Could you check a few things on this model? Use its own coordinates, in mm. A direction names the side the tool comes from. Round coordinates to 2 decimals unless told otherwise and drop trailing zeros. Write each loop counter-clockwise with the first axis right and the second up, starting at its lowest first coordinate (ties: lowest second). Pieces come first, ordered by that corner, then holes. Notation, with made-up numbers: (-31.5, 78) -> (-12.5, 78) arc R28 ccw to (-12.5, 112) -> close; hole circle Ø4 at (71, 82.25). An arc over 180 degrees is marked (long way). Answer in a Markdown table with one row per item.
from build123d import *

# Parameters (mm, degrees)
SHELL_1_T                = -4.4
SKETCH_4_W               = 30
SKETCH_4_H               = 20
CUT_EXTRUDE_2_DEPTH      = 143.273012367
FILLET_1_R               = 2
SKETCH_6_W               = 23
SKETCH_6_H               = 12.5
EXTRUDE_1_DEPTH          = 5.5
SKETCH_7_R               = 1.5
CUT_EXTRUDE_3_DEPTH      = 147.482115115
SKETCH_8_R               = 1.6
CUT_EXTRUDE_4_DEPTH      = 2.2
CUT_EXTRUDE_1_DEPTH      = 3.4
CUT_EXTRUDE_START        = -3.4
CUT_EXTRUDE_5_DEPTH      = 3.4
CUT_EXTRUDE_6_DEPTH      = 154.574086519
CUT_EXTRUDE_6_DEPTH_BACK = 154.574086519
SKETCH_10_R              = 2.75
SKETCH_11_R              = 3
EXTRUDE_2_DEPTH          = 3
HOLE_WIZARD_M3_1_D       = 3.4
HOLE_WIZARD_M3_1_DEPTH   = 4.4001
EXTRUDE_3_DEPTH          = 3


with BuildPart() as part:
    # 草图1 → 放样1 section 0
    with BuildSketch(Plane(origin=(0, 0, 0), x_dir=(1, 0, 0), z_dir=(0, 1, 0))):
        with BuildLine():
            Line((-62.5, 55), (62.5, 55))
            Line((62.5, 55), (62.5, -55))
            Line((62.5, -55), (-62.5, -55))
            Line((-62.5, -55), (-62.5, 55))
        make_face()
    # 草图2 → 放样1 section 1
    with BuildSketch(Plane(origin=(0, 72, 0), x_dir=(1, 0, 0), z_dir=(0, 1, 0))):
        with BuildLine():
            Line((-62.5, 55), (62.5, 55))
            Line((62.5, 55), (62.5, -55))
            Line((62.5, -55), (-62.5, -55))
            Line((-62.5, -55), (-62.5, 55))
        make_face()
    loft()

    # 抽壳1
    shell_1_openings = [part.faces().sort_by_distance(p)[0] for p in [
        (0, 72, 0),
    ]]
    offset(amount=SHELL_1_T, openings=shell_1_openings, kind=Kind.INTERSECTION)

    # 草图4 → 切除-拉伸2 (cut, through all)
    with BuildSketch(Plane.XY.offset(50.6)):
        with Locations((-22.217899847, 24.659135412)):
            Rectangle(SKETCH_4_W, SKETCH_4_H)
    extrude(amount=CUT_EXTRUDE_2_DEPTH, mode=Mode.SUBTRACT)

    # 圆角1
    fillet_1_edges = [part.edges().sort_by_distance(p)[0] for p in [
        (-7.217899847, 14.659135412, 52.8),
        (-7.217899847, 34.659135412, 52.8),
        (-37.217899847, 34.659135412, 52.8),
        (-37.217899847, 14.659135412, 52.8),
    ]]
    fillet(fillet_1_edges, radius=FILLET_1_R)

    # 草图6 → 凸台-拉伸1 (add)
    with BuildSketch(Plane(origin=(-58.1, 0, 0), x_dir=(0, 0, -1), z_dir=(1, 0, 0))):
        Polygon((-21.75, 42.25), (-21.75, 47.25), (11.25, 47.25), (11.25, 42.25), (11.25, 29.74999898), (11.25, 24.75), (-21.75, 24.75), (-21.75, 29.74999898), align=None)
        with Locations((-5.25, 36)):
            Rectangle(SKETCH_6_W, SKETCH_6_H, mode=Mode.SUBTRACT)
    extrude_1 = extrude(amount=EXTRUDE_1_DEPTH)

    # 草图7 → 切除-拉伸3 (cut, through all)
    with BuildSketch(Plane(origin=(-52.6, 0, 0), x_dir=(0, 0, -1), z_dir=(1, 0, 0))):
        with Locations(Location((-19, 35.99999884, 0), (0, 0, 90))):
            Circle(SKETCH_7_R)
        with Locations(Location((8.5, 35.99999884, 0), (0, 0, 90))):
            Circle(SKETCH_7_R)
    cut_extrude_3 = extrude(amount=-CUT_EXTRUDE_3_DEPTH, mode=Mode.SUBTRACT)

    # 镜向1: 凸台-拉伸1, 切除-拉伸3 across plane
    add(extrude_1.mirror(Plane(origin=(0, 0, 0), x_dir=(0, 0, 1), z_dir=(1, 0, 0))))
    add(cut_extrude_3.mirror(Plane(origin=(0, 0, 0), x_dir=(0, 0, 1), z_dir=(1, 0, 0))), mode=Mode.SUBTRACT)

    # 草图8 → 切除-拉伸4 (cut)
    with BuildSketch(Plane(origin=(0, 72, 0), x_dir=(1, 0, 0), z_dir=(0, 1, 0))):
        with Locations(Location((-60, 52.5, 0), (0, 0, 270))):
            Circle(SKETCH_8_R)
        with Locations(Location((-60, -52.5, 0), (0, 0, 270))):
            Circle(SKETCH_8_R)
        with Locations(Location((60, -52.5, 0), (0, 0, 270))):
            Circle(SKETCH_8_R)
        with Locations(Location((60, 52.5, 0), (0, 0, 270))):
            Circle(SKETCH_8_R)
    extrude(amount=-CUT_EXTRUDE_4_DEPTH, mode=Mode.SUBTRACT)

    # 草图3 → 切除-拉伸1 (cut)
    with BuildSketch(Plane(origin=(-58.1, 0, 0), x_dir=(0, 0, -1), z_dir=(1, 0, 0))):
        with BuildLine():
            ThreePointArc((-5.75, 38.449489743), (-8.75, 36), (-5.75, 33.550510257))
            ThreePointArc((-5.75, 33.550510257), (6.25, 36), (-5.75, 38.449489743))
        make_face()
    extrude(amount=-CUT_EXTRUDE_1_DEPTH, mode=Mode.SUBTRACT)

    # 草图9 → 切除-拉伸5 (cut)
    with BuildSketch(Plane.ZY.offset(-58.1).offset(CUT_EXTRUDE_START)):
        with BuildLine():
            ThreePointArc((5.75, 38.449489743), (-6.25, 36), (5.75, 33.550510257))
            ThreePointArc((5.75, 33.550510257), (8.75, 36), (5.75, 38.449489743))
        make_face()
    extrude(amount=CUT_EXTRUDE_5_DEPTH, mode=Mode.SUBTRACT)

    # 草图10 → 切除-拉伸6 (cut, two sides: drawn at the far end of the back side and taken through both)
    with BuildSketch(Plane(origin=(-61.5, 0, 0), x_dir=(0, 0, -1), z_dir=(1, 0, 0)).offset(-CUT_EXTRUDE_6_DEPTH_BACK)):
        with Locations(Location((0, 36, 0), (0, 0, 270))):
            Circle(SKETCH_10_R)
    extrude(amount=CUT_EXTRUDE_6_DEPTH + CUT_EXTRUDE_6_DEPTH_BACK, mode=Mode.SUBTRACT)

    # 草图11 → 凸台-拉伸2 (add)
    with BuildSketch(Plane(origin=(0, 0, -55), x_dir=(-1, 0, 0), z_dir=(0, 0, -1))):
        with Locations(Location((42.5, 24.543593294, 0), (0, 0, 270))):
            Circle(SKETCH_11_R)
        with Locations(Location((24.5, 24.543593294, 0), (0, 0, 270))):
            Circle(SKETCH_11_R)
    extrude(amount=EXTRUDE_2_DEPTH)

    # M3 间隙孔1
    with Locations(Plane(origin=(0, 0, 50.6), x_dir=(-1, 0, 0), z_dir=(0, 0, -1))):
        with Locations((-40.5, 63.5), (0, 63.5), (40.5, 63.5), (40.5, 36), (-40.5, 36)):
            Hole(HOLE_WIZARD_M3_1_D / 2, depth=HOLE_WIZARD_M3_1_DEPTH)

    # 草图15 → 凸台-拉伸3 (add)
    with BuildSketch(Plane(origin=(0, 0, 50.6), x_dir=(-1, 0, 0), z_dir=(0, 0, -1))):
        Polygon((-29.1, 60.00000762), (-29.1, 58), (-33.10001016, 58), (-33.10001016, 57), (-28.112700025, 57), (-28.1, 60.00000762), align=None)
        Polygon((-4.825356871, 58), (-4.825356871, 60.00000762), (-5.825356871, 60.00000762), (-5.825356871, 57.012700025), (-0.825346711, 57), (-0.825346711, 58), align=None)
        Polygon((-4.825356871, 32.025351791), (-0.825346711, 32.025351791), (-0.825346711, 33.025351791), (-5.825356871, 33.012651765), (-5.825356871, 30.025344171), (-4.825356871, 30.025344171), align=None)
        Polygon((-29.1, 32.025351791), (-29.1, 30.025344171), (-28.1, 30.025344171), (-28.1, 33.012651765), (-28.1, 33.025351791), (-33.10001016, 33.025351791), (-33.10001016, 32.025351791), align=None)
    extrude(amount=EXTRUDE_3_DEPTH)


solid = part.part
1) For faces 1 (the face through (-43, 25, -58)), 2 (the face through (-22, 34.659, 53)), 3 (the face through (-58.1, 31, -5)), 4 (the face through (61.35, 70.92, 53.36)), 5 (the face through (-62.5, 29, 1)), which set-ups out of +Z, -Z, +X, -X, +Y, -Y let a thin tool reach every point of the face, with its end or its side?
Findings:
| item | result |
|---|---|
| face 1 | -Z, +X, -X, +Y, -Y |
| face 2 | +Z |
| face 3 | none |
| face 4 | +Y |
| face 5 | +Z, -Z, -X, +Y, -Y |
2) Imagine slicing it at A-A, the plane x = -24.5. Please give me the cut outline in (y, z), plus the area to 3 significant figures.
Findings:
| item | result |
|---|---|
| outline | (0, -55) -> (21.54, -55) -> (21.54, -58) -> (27.54, -58) -> (27.54, -55) -> (72, -55) -> (72, -50.6) -> (4.4, -50.6) -> (4.4, 50.6) -> (14.66, 50.6) -> (14.66, 55) -> (0, 55) -> close; (34.66, 50.6) -> (72, 50.6) -> (72, 55) -> (34.66, 55) -> close |
| area | 1,010 mm^2 |
3) Thinking about a two-plate mould opening in Y: for faces 6 (the face through (52.6, 44, 5)), 7 (the face through (55, 47.25, 5)), 8 (the face through (55, 36, -6.25)), which applies, +Y half, -Y half, draft (parallel to the pull), parting line (faces both ways), or undercut?
Findings:
| item | result |
|---|---|
| face 6 | draft |
| face 7 | +Y half |
| face 8 | undercut |
4) For pin 1 (18 mm diameter, centred on y = 34.5, z = 0.5, fed in from +X); pin 2 (3 mm diameter, centred on x = -9.5, z = -28, fed in from +Y); pin 3 (3 mm diameter, centred on x = -28.5, y = 55.5, fed in from -Z); pin 4 (0.8 mm diameter, centred on x = 5.5, z = 48.5, fed in from +Y), each with a flat end and sliding along its axis, tell me the tip position at first contact or that it passes through.
Findings:
| item | result |
|---|---|
| pin 1 | stops at x = 62.5 |
| pin 2 | stops at y = 4.4 |
| pin 3 | stops at z = -55 |
| pin 4 | stops at y = 60 |
5) Please list where these lines run through material, in increasing order: line 1 (Y direction, x = -40.5, z = 54); line 2 (Z direction, x = 53, y = 30.5); line 3 (Z direction, x = -56, y = 49).
Findings:
| item | result |
|---|---|
| line 1 | y = 0 to 34.3, 37.7 to 61.8, 65.2 to 72 |
| line 2 | z = -55 to -50.6, -11.25 to -6.25, 16.75 to 21.75, 50.6 to 55 |
| line 3 | z = -55 to -50.6, 50.6 to 55 |
6) Imagine slicing it at C-C, the plane y = 63.5. Please give me the cut outline in (x, z).
Findings:
| item | result |
|---|---|
| outline | (-62.5, -55) -> (62.5, -55) -> (62.5, 55) -> (42.2, 55) -> (42.2, 50.6) -> (58.1, 50.6) -> (58.1, -50.6) -> (-58.1, -50.6) -> (-58.1, 50.6) -> (-42.2, 50.6) -> (-42.2, 55) -> (-62.5, 55) -> close; (-38.8, 50.6) -> (-1.7, 50.6) -> (-1.7, 55) -> (-38.8, 55) -> close; (1.7, 50.6) -> (38.8, 50.6) -> (38.8, 55) -> (1.7, 55) -> close |
7) Imagine slicing it at D-D, the plane x = -48. Please give me the cut outline in (y, z), plus the area to 3 significant figures.
Findings:
| item | result |
|---|---|
| outline | (0, -55) -> (72, -55) -> (72, -50.6) -> (4.4, -50.6) -> (4.4, 50.6) -> (72, 50.6) -> (72, 55) -> (0, 55) -> close |
| area | 1,080 mm^2 |
8) Imagine slicing it at B-B, the plane z = 19. Please give me the cut outline in (x, y), plus the area to 3 significant figures.
Findings:
| item | result |
|---|---|
| outline | (-62.5, 0) -> (62.5, 0) -> (62.5, 34.5) -> (52.6, 34.5) -> (52.6, 24.75) -> (58.1, 24.75) -> (58.1, 4.4) -> (-58.1, 4.4) -> (-58.1, 24.75) -> (-52.6, 24.75) -> (-52.6, 34.5) -> (-62.5, 34.5) -> close; (-62.5, 37.5) -> (-52.6, 37.5) -> (-52.6, 47.25) -> (-58.1, 47.25) -> (-58.1, 72) -> (-62.5, 72) -> close; (52.6, 37.5) -> (62.5, 37.5) -> (62.5, 72) -> (58.1, 72) -> (58.1, 47.25) -> (52.6, 47.25) -> close |
| area | 1,330 mm^2 |
